Part model, mm, in its own coordinate system. Face numbers are marked on the shaded views. Give positions to 0.01 mm unless a question says otherwise; leave off trailing zeros. Order: outer loops, then holes, each group sorted by start corner. A loop starts at its lowest first (then second) coordinate and runs counter-clockwise, first axis right, second up. Notation, with made-up numbers: (45, -19) -> (79, -19) arc R34 cw to (79, 20) -> close; hole circle Ø6 at (18.25, -25.5). An arc over 180 degrees is marked (long way). Write item = value, one per line. Start each with the question number.
Item 1: Pull direction Z, two halves, no side cores. Call the marked faces 1, 2, 3 and 4: +Z half, -Z half, draft (parallel to the pull), parting line (faces both ways), or undercut.
Item 2: Band-saw the part on A-A on y = 6. Write the cut outline in (x, z), plus the area to 3 significant figures.
Item 3: Drill centre lines: line 1 along Z through (x, y) = (7, 4.1); line 2 along X through (y, z) = (2.95, 6.5); line 3 along Y through (x, z) = (59, 9.25). Where is each one in solid material? Low to high.
Item 4: Band-saw the part on C-C on x = -7. Write the cut outline in (y, z), plus the area to 3 significant figures.
Item 5: Band-saw the part on D-D on x = 67. Write the cut outline in (y, z), plus the area to 3 significant figures.
Item 6: Flat gauge pins, fed straight in: P1, Ø1.8, axis at y = 4.5, z = -3, coming from the -X side; P2, Ø0.9, axis at x = -1.5, y = 4, coming from the -Z side; P3, Ø6, axis at x = 59.5, y = 4, coming from the +Z side. Where does each tip first touch, or does it go through?
Item 7: Band-saw the part on B-B on z = 2.25. Write the cut outline in (x, y), plus the area to 3 significant figures.
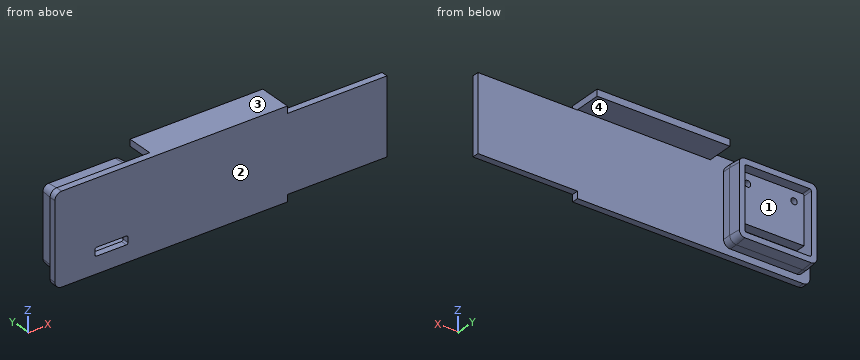
```python
from build123d import *
from OCP.BRepFilletAPI import BRepFilletAPI_MakeChamfer

# Parameters (mm, degrees)
SKETCH1_W           = 28
SKETCH1_H           = 27
BOSS_EXTRUDE1_DEPTH = 2
SKETCH2_W           = 10
SKETCH2_H           = 2.5
CUT_EXTRUDE1_DEPTH  = 2
SKETCH3_W           = 20
SKETCH3_H           = 14.5
BOSS_EXTRUDE2_DEPTH = 3
SKETCH4_W           = 24
SKETCH4_H           = 23
SKETCH4_W_2         = 20
SKETCH4_H_2         = 19
BOSS_EXTRUDE3_DEPTH = 6
SKETCH5_R           = 0.95
CUT_EXTRUDE2_DEPTH  = 3.2
FILLET3_R           = 2
FILLET2_R           = 0.5
SKETCH6_W           = 27
SKETCH6_H           = 2
BOSS_EXTRUDE4_DEPTH = 72
CHAMFER1_SIZE       = 3.5
CHAMFER1_SIZE2      = 0.306210322
SKETCH7_W           = 30
SKETCH7_H           = 2.1
CUT_EXTRUDE3_DEPTH  = 88.259669951
SKETCH8_W           = 40
SKETCH8_H           = 8
BOSS_EXTRUDE5_DEPTH = 2


with BuildPart() as part:
    # Sketch1 → Boss-Extrude1 (new body)
    with BuildSketch(Plane(origin=(0, 0, 0), x_dir=(1, 0, 0), z_dir=(0, 1, 0))):
        Rectangle(SKETCH1_W, SKETCH1_H)
    extrude(amount=BOSS_EXTRUDE1_DEPTH)

    # Sketch2 → Cut-Extrude1 (cut)
    with BuildSketch(Plane(origin=(0, 2, 0), x_dir=(1, 0, 0), z_dir=(0, 1, 0))):
        with Locations((3, 7.25)):
            Rectangle(SKETCH2_W, SKETCH2_H)
    extrude(amount=-CUT_EXTRUDE1_DEPTH, mode=Mode.SUBTRACT)

    # Sketch3 → Boss-Extrude2 (add)
    with BuildSketch(Plane(origin=(0, 2, 0), x_dir=(1, 0, 0), z_dir=(0, 1, 0))):
        with Locations((0, -2.25)):
            Rectangle(SKETCH3_W, SKETCH3_H)
    extrude(amount=BOSS_EXTRUDE2_DEPTH)

    # Sketch4 → Boss-Extrude3 (add)
    with BuildSketch(Plane(origin=(0, 2, 0), x_dir=(1, 0, 0), z_dir=(0, 1, 0))):
        Rectangle(SKETCH4_W, SKETCH4_H)
        Rectangle(SKETCH4_W_2, SKETCH4_H_2, mode=Mode.SUBTRACT)
    extrude(amount=BOSS_EXTRUDE3_DEPTH)

    # Sketch5 → Cut-Extrude2 (cut)
    with BuildSketch(Plane(origin=(0, 5, 0), x_dir=(1, 0, 0), z_dir=(0, 1, 0))):
        with Locations(Location((-7, -6.5, 0), (0, 0, 270))):
            Circle(SKETCH5_R)
        with Locations(Location((7, -6.5, 0), (0, 0, 90))):
            Circle(SKETCH5_R)
    extrude(amount=-CUT_EXTRUDE2_DEPTH, mode=Mode.SUBTRACT)

    # Fillet3
    fillet3_edges = [part.edges().sort_by_distance(p)[0] for p in [
        (12, 5, -11.5),
        (-12, 5, -11.5),
        (-12, 5, 11.5),
        (12, 5, 11.5),
        (-14, 1, 13.5),
        (-14, 1, -13.5),
    ]]
    fillet(fillet3_edges, radius=FILLET3_R)

    # Fillet2
    fillet2_edges = [part.edges().sort_by_distance(p)[0] for p in [
        (-2, 1, -8.5),
        (-2, 1, -6),
        (8, 1, -6),
        (8, 1, -8.5),
        (10, 5, -9.5),
        (-10, 6.5, 9.5),
        (10, 6.5, 9.5),
        (-10, 5, -9.5),
    ]]
    fillet(fillet2_edges, radius=FILLET2_R)

    # Sketch6 → Boss-Extrude4 (add)
    with BuildSketch(Plane(origin=(14, 0, 0), x_dir=(0, 0, -1), z_dir=(1, 0, 0))):
        with Locations((0, 1)):
            Rectangle(SKETCH6_W, SKETCH6_H)
    extrude(amount=BOSS_EXTRUDE4_DEPTH)

    # Chamfer1: one chamfer whose edges measure the first distance from different faces: ONE call of the kernel's chamfer builder (chamfer() names one face for all edges)
    chamfer1_edges_1 = [part.edges().sort_by_distance(p)[0] for p in [
        (0, 8, -11.5),
    ]]
    chamfer1_side_1 = [part.faces().sort_by_distance(p)[0] for p in [
        (0, 5, -11.5),
    ]]
    chamfer1_edges_2 = [part.edges().sort_by_distance(p)[0] for p in [
        (12, 8, 0),
    ]]
    chamfer1_side_2 = [part.faces().sort_by_distance(p)[0] for p in [
        (12, 5, 0),
    ]]
    chamfer1_edges_3 = [part.edges().sort_by_distance(p)[0] for p in [
        (-12, 8, 0),
    ]]
    chamfer1_side_3 = [part.faces().sort_by_distance(p)[0] for p in [
        (-12, 5, 0),
    ]]
    chamfer1_edges_4 = [part.edges().sort_by_distance(p)[0] for p in [
        (0, 8, 11.5),
    ]]
    chamfer1_side_4 = [part.faces().sort_by_distance(p)[0] for p in [
        (0, 5, 11.5),
    ]]
    chamfer1_edges_5 = [part.edges().sort_by_distance(p)[0] for p in [
        (-11.414213562, 8, -10.914213562),
    ]]
    chamfer1_side_5 = [part.faces().sort_by_distance(p)[0] for p in [
        (-11.414213562, 5, -10.914213562),
    ]]
    chamfer1_edges_6 = [part.edges().sort_by_distance(p)[0] for p in [
        (-11.414213562, 8, 10.914213562),
    ]]
    chamfer1_side_6 = [part.faces().sort_by_distance(p)[0] for p in [
        (-11.414213562, 5, 10.914213562),
    ]]
    chamfer1_edges_7 = [part.edges().sort_by_distance(p)[0] for p in [
        (11.414213562, 8, 10.914213562),
    ]]
    chamfer1_side_7 = [part.faces().sort_by_distance(p)[0] for p in [
        (11.414213562, 5, 10.914213562),
    ]]
    chamfer1_edges_8 = [part.edges().sort_by_distance(p)[0] for p in [
        (11.414213562, 8, -10.914213562),
    ]]
    chamfer1_side_8 = [part.faces().sort_by_distance(p)[0] for p in [
        (11.414213562, 5, -10.914213562),
    ]]
    chamfer1 = BRepFilletAPI_MakeChamfer(part.part.solid().wrapped)
    for e in chamfer1_edges_1:
        chamfer1.Add(CHAMFER1_SIZE, CHAMFER1_SIZE2, e.wrapped, chamfer1_side_1[0].wrapped)  # the first distance lies on this face
    for e in chamfer1_edges_2:
        chamfer1.Add(CHAMFER1_SIZE, CHAMFER1_SIZE2, e.wrapped, chamfer1_side_2[0].wrapped)  # the first distance lies on this face
    for e in chamfer1_edges_3:
        chamfer1.Add(CHAMFER1_SIZE, CHAMFER1_SIZE2, e.wrapped, chamfer1_side_3[0].wrapped)  # the first distance lies on this face
    for e in chamfer1_edges_4:
        chamfer1.Add(CHAMFER1_SIZE, CHAMFER1_SIZE2, e.wrapped, chamfer1_side_4[0].wrapped)  # the first distance lies on this face
    for e in chamfer1_edges_5:
        chamfer1.Add(CHAMFER1_SIZE, CHAMFER1_SIZE2, e.wrapped, chamfer1_side_5[0].wrapped)  # the first distance lies on this face
    for e in chamfer1_edges_6:
        chamfer1.Add(CHAMFER1_SIZE, CHAMFER1_SIZE2, e.wrapped, chamfer1_side_6[0].wrapped)  # the first distance lies on this face
    for e in chamfer1_edges_7:
        chamfer1.Add(CHAMFER1_SIZE, CHAMFER1_SIZE2, e.wrapped, chamfer1_side_7[0].wrapped)  # the first distance lies on this face
    for e in chamfer1_edges_8:
        chamfer1.Add(CHAMFER1_SIZE, CHAMFER1_SIZE2, e.wrapped, chamfer1_side_8[0].wrapped)  # the first distance lies on this face
    add(Compound.cast(chamfer1.Shape()), mode=Mode.REPLACE)

    # Sketch7 → Cut-Extrude3 (cut, through all)
    with BuildSketch(Plane(origin=(0, 2, 0), x_dir=(1, 0, 0), z_dir=(0, 1, 0))):
        with Locations((71, 12.45)):
            Rectangle(SKETCH7_W, SKETCH7_H)
    cut_extrude3 = extrude(amount=-CUT_EXTRUDE3_DEPTH, mode=Mode.SUBTRACT)

    # Mirror1: Cut-Extrude3 across plane
    add(cut_extrude3.mirror(Plane.XY), mode=Mode.SUBTRACT)

    # Sketch8 → Boss-Extrude5 (add)
    with BuildSketch(Plane.XY.offset(13.5)):
        with Locations((36, 6)):
            Rectangle(SKETCH8_W, SKETCH8_H)
    extrude(amount=-BOSS_EXTRUDE5_DEPTH)


solid = part.part
```
Values found:
q1.face_1 = undercut
q1.face_2 = draft
q1.face_3 = +Z half
q1.face_4 = -Z half
q2.outline = (-11.87, -9.5) arc R1.87 ccw to (-10, -11.37) -> (10, -11.37) arc R1.87 ccw to (11.87, -9.5) -> (11.87, 9.5) arc R1.87 ccw to (10, 11.37) -> (-10, 11.37) arc R1.87 ccw to (-11.87, 9.5) -> close; (16, 11.5) -> (56, 11.5) -> (56, 13.5) -> (16, 13.5) -> close; hole (-10, -9) arc R0.5 ccw to (-9.5, -9.5) -> (9.5, -9.5) arc R0.5 ccw to (10, -9) -> (10, 9) arc R0.5 ccw to (9.5, 9.5) -> (-9.5, 9.5) arc R0.5 ccw to (-10, 9) -> close
q2.area = 237 mm^2
q3.line_1 = -11.5 to -9.5, -5 to 5.55, 7.45 to 11.5
q3.line_2 = -12 to -7.95, -6.05 to 6.05, 7.95 to 12
q3.line_3 = 0 to 2
q4.outline = (0, -13.5) -> (2, -13.5) -> (2, -11.5) -> (4.5, -11.5) -> (8, -11.19) -> (8, -9.5) -> (2, -9.5) -> (2, -5) -> (5, -5) -> (5, 5.55) -> (1.8, 5.55) -> (1.8, 7.45) -> (5, 7.45) -> (5, 9.5) -> (8, 9.5) -> (8, 11.19) -> (4.5, 11.5) -> (2, 11.5) -> (2, 13.5) -> (0, 13.5) -> close
q4.area = 114 mm^2
q5.outline = (0, -11.4) -> (2, -11.4) -> (2, 11.4) -> (0, 11.4) -> close
q5.area = 45.6 mm^2
q6.P1 = -12
q6.P2 = -11.5
q6.P3 = 11.4
q7.outline = (-14, 0) -> (86, 0) -> (86, 2) -> (12, 2) -> (12, 4.5) -> (11.69, 8) -> (10, 8) -> (10, 5) -> (-10, 5) -> (-10, 8) -> (-11.69, 8) -> (-12, 4.5) -> (-12, 2) -> (-14, 2) -> close
q7.area = 283 mm^2
